Could you check a few things on this model? Use its own coordinates, in mm. A direction names the side the tool comes from. Coordinates: 2 decimals unless noted, no trailing zeros. Loops run counter-clockwise (first coordinate to the right, second up) from the corner with the lowest first, then second, coordinate; pieces in that order, holes last.
1) Imagine slicing it at C-C on y = 19.05. Please give me the cut outline in (x, z) (3 decimals), plus the area to 3 significant figures.
2) Will these pins go through, and if not, where does the flat tip stop? P1, Ø19, axis at x = 16, y = 14.5, coming from the +Z side; P2, Ø5, axis at x = 34, z = 102.5, coming from the -Y side.
3) For faces 1 (the face through (37.41, 15.95, 94.81)), 2 (the face through (24, 19, 60.325)), 3 (the face through (19.693, 36.49, 15.213)), which set-ups out of +Z, -Z, +X, -X, +Y, -Y let a thin tool reach every point of the face, with its end or its side?
4) If I drill on line 1 along Y through (x, z) = (27.5, 31.5) (3 decimals); line 2 along Z through (x, y) = (26.5, 35); line 3 along Z through (x, y) = (36.5, 15.5) (3 decimals), over which ranges is the centre line in solid material (lowest first)?
5) Imagine slicing it at B-B on x = 12.5. Please give me the cut outline in (y, z) (3 decimals), plus the area to 3 significant figures.
6) Imagine slicing it at A-A on z = 58. Please give me the cut outline in (x, y) (3 decimals).
7) Imagine slicing it at D-D on x = 23.5. Please give me the cut outline in (y, z) (3 decimals).
8) Thinking about a two-plate mould opening in Y: for faces 4 (the face through (24, 34.925, 30)), 5 (the face through (24, 3.175, 30)), 6 (the face through (23, 37, 0)), 7 (the face through (23, 0, 31)), which applies, released by +Y, released by -Y, zero draft, split by the parting line, or undercut?
```python
from build123d import *

# Parameters (mm, degrees)
F0_W     = 47.625
F0_H     = 38.1
F1_DEPTH = 63.5
F2_W     = 31.75
F2_H     = 60.325
F3_DEPTH = 47.625
F4_R     = 3.175
F5_DEPTH = 63.5
F6_R     = 3.175
F7_DEPTH = 45.974


with BuildPart() as f1:
    # F0 (on Top) → F1 (new body)
    with BuildSketch(Plane.XY):
        with Locations((23.8125, 19.05)):
            Rectangle(F0_W, F0_H)
    extrude(amount=F1_DEPTH)

    # F2 (on face) → F3 (cut)
    with BuildSketch(Plane.YZ.offset(47.625)):
        with Locations((19.05, 30.1625)):
            Rectangle(F2_W, F2_H)
    extrude(amount=-F3_DEPTH, mode=Mode.SUBTRACT)

    # F4 (on face) → F5 (join)
    with BuildSketch(Plane.XY.offset(63.5)):
        with Locations((38.1, 19.05)):
            Circle(F4_R)
    extrude(amount=F5_DEPTH)

    # F6 (on face) → F7 (cut)
    with BuildSketch(Plane.XZ):
        with Locations((22.212138, 17.145)):
            Circle(F6_R)
    extrude(amount=-F7_DEPTH, mode=Mode.SUBTRACT)


solid = f1.part
```
Filled in:
1. outline: (0, 60.325) - (47.625, 60.325) - (47.625, 63.5) - (41.275, 63.5) - (41.275, 127) - (34.925, 127) - (34.925, 63.5) - (0, 63.5) - close
1. area: 554 mm2
2. P1: stops at z = 63.5
2. P2: stops at y = 16.31
3. face 1: +Z
3. face 2: -Z, +X, -X
3. face 3: +Y, -Y
4. line 1: y = 0 to 3.175, 34.925 to 38.1
4. line 2: z = 0 to 63.5
4. line 3: z = 60.325 to 63.5
5. outline: (0, 0) - (3.175, 0) - (3.175, 60.325) - (34.925, 60.325) - (34.925, 0) - (38.1, 0) - (38.1, 63.5) - (0, 63.5) - close
5. area: 504 mm2
6. outline: (0, 0) - (47.625, 0) - (47.625, 3.175) - (0, 3.175) - close; (0, 34.925) - (47.625, 34.925) - (47.625, 38.1) - (0, 38.1) - close
7. outline: (0, 0) - (3.175, 0) - (3.175, 14.243) - (0, 14.243) - close; (0, 20.047) - (3.175, 20.047) - (3.175, 60.325) - (34.925, 60.325) - (34.925, 20.047) - (38.1, 20.047) - (38.1, 63.5) - (0, 63.5) - close; (34.925, 0) - (38.1, 0) - (38.1, 14.243) - (34.925, 14.243) - close
8. face 4: undercut
8. face 5: undercut
8. face 6: zero draft
8. face 7: released by -Y
